from build123d import *

# Parameters (mm, degrees)
F0_W     = 101.6
F0_H     = 76.2
F1_DEPTH = 25.4
F3_D     = 63.5
F5_DEPTH = 25.4


with BuildPart() as f1:
    # F0 (on Front) → F1 (new body)
    with BuildSketch(Plane.XZ):
        with Locations((50.8, 38.1)):
            Rectangle(F0_W, F0_H)
    extrude(amount=F1_DEPTH)

    # F3 (through all)
    with Locations(Plane.XZ.offset(25.4)):
        with Locations((51.822923, 34.358785)):
            Hole(F3_D / 2)

    # F4 (on face) → F5 (join)
    with BuildSketch(Plane.XY.offset(76.2)):
        Polygon((61.826725, -3.606968), (57.771097, -7.324631), (60.053547, -12.330584), (65.519807, -11.706769), (66.615691, -6.315278), align=None)
    extrude(amount=F5_DEPTH)


solid = f1.part
The model under review builds one solid part; all positions refer to its coordinate system, in mm. A direction names the side the tool comes from. Coordinates: 2 decimals unless noted, no trailing zeros. Loops run counter-clockwise (first coordinate to the right, second up) from the corner with the lowest first, then second, coordinate; pieces in that order, holes last. Notation, with made-up numbers: M 62.5,21.5 L 71.5,21.5 A20 cw 71.5,52.5 Z; hole C 6.25,-33 d5. An arc over 180 degrees is marked long. Put each result on its own line as item: value. Start each with the question number.
Q1. Add section D-D (z = 93.5). Write out the cut boundary in (x, y), and give its area (3 significant figures).
Q2. Add section A-A (z = 59.5). Write out the cut boundary in (x, y), and give its area (3 significant figures).
Q3. For faces 1 (the flat face through (50, -13, 0)), 2 (the flat face through (66.06, -9.05, 88.72)), 3 (the flat face through (59.83, -5.44, 88.72)), list the 3-axis set-ups (+Z, -Z, +X, -X, +Y, -Y) from which the entire face can be reached by the end or side of a thin tool; tool diameter is ignored.
Q4. Wall thickness on line 1 (Z direction, x = 79, y = -9.5); line 2 (X direction, y = -21.75, z = 63.5); line 3 (Z direction, x = 24, y = -19): over which ranges is each line inside the solid? List them lowest first.
Q5. Add section B-B (x = 30.5). Write out the cut boundary in (y, z), and give its area (3 significant figures).
Q6. Clearance check with a flat-ended pin moving along its axis: pin 1 (12.5 mm diameter, centred on x = 40, y = -13.5, fed in from +Z). State where the tip first meets the part, or that it passes through.
Q7. The part is to be moulded in two halves that separate along X. For faces 4 (the cylindrical face through (58.706, -12.522, 3.364)), 5 (the flat face through (64.255, -4.98, 88.722)), 6 (the flat face through (58.9, -9.8, 88.7)), say which applies: +X half, -X half, draft (parallel to the pull), parting line (faces both ways), or undercut.
Q8. Add section C-C (y = -10.5). Write out the cut boundary in (x, z), and give its area (3 significant figures).
Answers:
1. outline: M 57.77,-7.32 L 60.05,-12.33 L 65.52,-11.71 L 66.62,-6.32 L 61.83,-3.61 Z
1. area: 52.1 mm^2
2. outline: M 0,-25.4 L 32.43,-25.4 L 32.43,0 L 0,0 Z; M 71.21,-25.4 L 101.6,-25.4 L 101.6,0 L 71.21,0 Z
2. area: 1,600 mm^2
3. face 1: -Z, +X, -X, +Y, -Y
3. face 2: +Z, +X, -Y
3. face 3: +Z, -X, +Y
4. line 1: z = 0 to 17.94, 50.77 to 76.2
4. line 2: x = 0 to 39.22, 64.43 to 101.6
4. line 3: z = 0 to 19.06, 49.65 to 76.2
5. outline: M -25.4,0 L 0,0 L 0,10.83 L -25.4,10.83 Z; M -25.4,57.88 L 0,57.88 L 0,76.2 L -25.4,76.2 Z
5. area: 740 mm^2
6. pin 1: stops at z = 76.2
7. face 4: undercut
7. face 5: +X half
7. face 6: -X half
8. outline: M 0,0 L 101.6,0 L 101.6,76.2 L 65.77,76.2 L 65.77,101.6 L 59.22,101.6 L 59.22,76.2 L 0,76.2 Z; hole C 51.82,34.36 d63.5
8. area: 4,740 mm^2
